from build123d import *

# Parameters (mm, degrees)
SKETCH1_W           = 120
SKETCH1_H           = 200
SKETCH1_R           = 1.65
SKETCH1_W_2         = 3
SKETCH1_H_2         = 20
SKETCH1_W_3         = 20
SKETCH1_H_3         = 3
BOSS_EXTRUDE1_DEPTH = 3


with BuildPart() as part:
    # Sketch1 → Boss-Extrude1 (new body)
    with BuildSketch(Plane.XY):
        with Locations((-8.436124494, -75.291436911)):
            Rectangle(SKETCH1_W, SKETCH1_H)
        with Locations((-55.436124494, 14.708563089)):
            Circle(SKETCH1_R, mode=Mode.SUBTRACT)
        with Locations((-15.436124494, 14.708563089)):
            Circle(SKETCH1_R, mode=Mode.SUBTRACT)
        with Locations((-15.436124494, -25.291436911)):
            Circle(SKETCH1_R, mode=Mode.SUBTRACT)
        with Locations((-55.436124494, -25.291436911)):
            Circle(SKETCH1_R, mode=Mode.SUBTRACT)
        with Locations((-0.436547566, 14.821221739)):
            Circle(SKETCH1_R, mode=Mode.SUBTRACT)
        with Locations((39.563452434, 14.821221739)):
            Circle(SKETCH1_R, mode=Mode.SUBTRACT)
        with Locations((39.563452434, -25.178778261)):
            Circle(SKETCH1_R, mode=Mode.SUBTRACT)
        with Locations((-0.436547566, -25.178778261)):
            Circle(SKETCH1_R, mode=Mode.SUBTRACT)
        with Locations((-53.436124494, -75.291436911)):
            Circle(SKETCH1_R, mode=Mode.SUBTRACT)
        with Locations((25.563875506, -75.291436911)):
            Circle(SKETCH1_R, mode=Mode.SUBTRACT)
        with Locations((25.563875506, -141.591436911)):
            Circle(SKETCH1_R, mode=Mode.SUBTRACT)
        with Locations((-53.436124494, -141.591436911)):
            Circle(SKETCH1_R, mode=Mode.SUBTRACT)
        with Locations((-51.436124494, -170.291436911)):
            Circle(SKETCH1_R, mode=Mode.SUBTRACT)
        with Locations((35.063875506, 20.708563089)):
            Circle(SKETCH1_R, mode=Mode.SUBTRACT)
        with Locations((-65.436124494, -25.291436911)):
            Rectangle(SKETCH1_W_2, SKETCH1_H_2, mode=Mode.SUBTRACT)
        with Locations((-65.436124494, -75.291436911)):
            Rectangle(SKETCH1_W_2, SKETCH1_H_2, mode=Mode.SUBTRACT)
        with Locations((-65.436124494, -125.291436911)):
            Rectangle(SKETCH1_W_2, SKETCH1_H_2, mode=Mode.SUBTRACT)
        with Locations((48.563875506, -25.291436911)):
            Rectangle(SKETCH1_W_2, SKETCH1_H_2, mode=Mode.SUBTRACT)
        with Locations((48.563875506, -75.291436911)):
            Rectangle(SKETCH1_W_2, SKETCH1_H_2, mode=Mode.SUBTRACT)
        with Locations((48.563875506, -125.291436911)):
            Rectangle(SKETCH1_W_2, SKETCH1_H_2, mode=Mode.SUBTRACT)
        with Locations((-38.436124494, -172.291436911)):
            Rectangle(SKETCH1_W_3, SKETCH1_H_3, mode=Mode.SUBTRACT)
        with Locations((-8.436124494, -172.291436911)):
            Rectangle(SKETCH1_W_3, SKETCH1_H_3, mode=Mode.SUBTRACT)
        with Locations((21.563875506, -172.291436911)):
            Rectangle(SKETCH1_W_3, SKETCH1_H_3, mode=Mode.SUBTRACT)
        with Locations((-38.436124494, 21.708563089)):
            Rectangle(SKETCH1_W_3, SKETCH1_H_3, mode=Mode.SUBTRACT)
        with Locations((-8.436124494, 21.708563089)):
            Rectangle(SKETCH1_W_3, SKETCH1_H_3, mode=Mode.SUBTRACT)
        with Locations((21.563875506, 21.708563089)):
            Rectangle(SKETCH1_W_3, SKETCH1_H_3, mode=Mode.SUBTRACT)
    extrude(amount=BOSS_EXTRUDE1_DEPTH)


solid = part.part
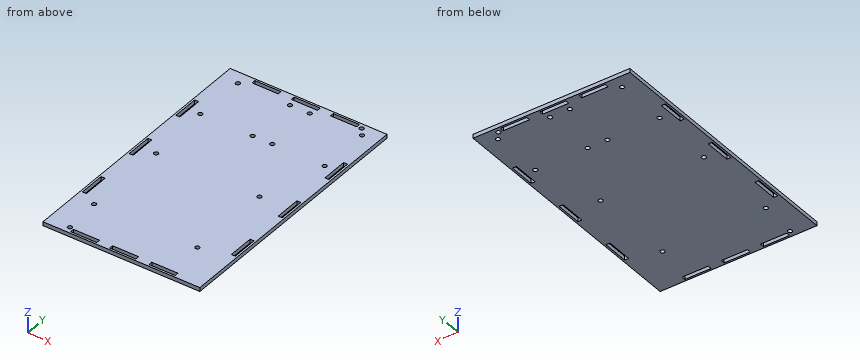
Work out the finished part from the listing and answer in its coordinate system (mm). Round coordinates to 2 decimals unless told otherwise and drop trailing zeros. Loops run counter-clockwise (first coordinate to the right, second up) from the corner with the lowest first, then second, coordinate; pieces in that order, holes last. Notation, with made-up numbers: (-11, 34.25) -> (10, 34.25) arc R19 cw to (10, 57.25) -> close; hole circle Ø1 at (52.5, 11.5). An arc over 180 degrees is marked (long way). Use one line per item in the form item = value.
(1) Find section A-A on y = -83. Give the vertices of the cut face in (x, z).
Answer list:
outline = (-68.44, 0) -> (-66.94, 0) -> (-66.94, 3) -> (-68.44, 3) -> close; (-63.94, 0) -> (47.06, 0) -> (47.06, 3) -> (-63.94, 3) -> close; (50.06, 0) -> (51.56, 0) -> (51.56, 3) -> (50.06, 3) -> close
(2) Straight lines are drawn through the part: line 1 (Y direction, x = 23.5, z = 2.15); line 2 (X direction, y = -115.5, z = 2.4); line 3 (Y direction, x = 0, z = 1.1). For each, find the intervals that lie inside material, in ascending order.
Answer list:
line_1 = -175.29 to -173.79, -170.79 to 20.21, 23.21 to 24.71
line_2 = -68.44 to -66.94, -63.94 to 47.06, 50.06 to 51.56
line_3 = -175.29 to -173.79, -170.79 to -26.77, -23.59 to 13.23, 16.41 to 20.21, 23.21 to 24.71
(3) Find section C-C on z = 1.25. Give the number of separate pieces and of enclosed holes in the cut face, then the cut area to 3 significant figures.
Answer list:
separate_pieces = 1
enclosed_holes = 26
area = 23,200 mm2
(4) Find section B-B on x = 15. Give the vertices of the cut face in (y, z).
Answer list:
outline = (-175.29, 0) -> (-173.79, 0) -> (-173.79, 3) -> (-175.29, 3) -> close; (-170.79, 0) -> (20.21, 0) -> (20.21, 3) -> (-170.79, 3) -> close; (23.21, 0) -> (24.71, 0) -> (24.71, 3) -> (23.21, 3) -> close
